Check sheet for the modelled part. Datum: model origin and axes. Units: mm. Face numbers are marked on the shaded views. A direction names the side the tool comes from. Round coordinates to 2 decimals unless told otherwise and drop trailing zeros. Order: outer loops, then holes, each group sorted by start corner. A loop starts at its lowest first (then second) coordinate and runs counter-clockwise, first axis right, second up. Notation, with made-up numbers: (85, -22.75) -> (140, -22.75) arc R10 ccw to (140, -14.75) -> close; hole circle Ø8 at (84.25, -8.5). An arc over 180 degrees is marked (long way). Answer in a Markdown table with one row per item.
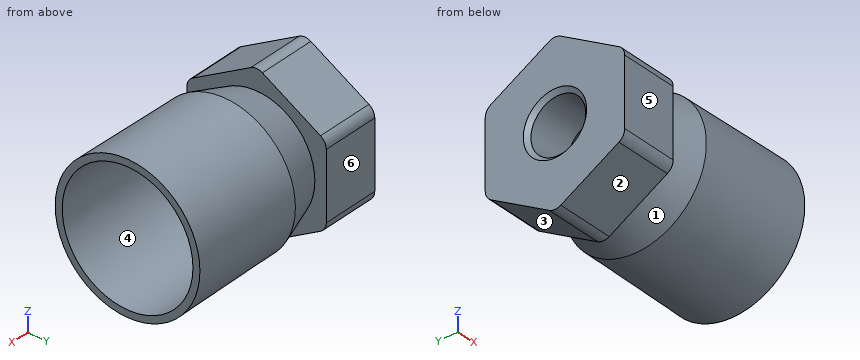
Autodesk Inventor part; units mm, degrees
ref_plane "YZ Plane" through (0, 0, 0) normal (1, 0, 0) x (0, 1, 0)
ref_plane "XZ Plane" through (0, 0, 0) normal (0, 1, 0) x (-1, 0, 0)
ref_plane "XY Plane" through (0, 0, 0) normal (0, 0, 1) x (1, 0, 0)
sketch "Sketch1" plane through (0, 0, 0) normal (0, 0, 1) x (1, 0, 0)
  line L0 (0, 0) -> (6.6144, 0) construction
  line L1 (0, 0) -> (0, 4.75) construction
  line L2 (0, 4.75) -> (8, 4.3864)
  line L3 (6.6144, 0) -> (16.6144, 0) construction
  line L4 (16.6144, 0) -> (16.6144, 12.2) construction
  line L5 (16.6144, 0) -> (36.6144, 0) construction
  line L6 (36.6144, 0) -> (36.6144, 12.45) construction
  line L7 (36.6144, 12.45) -> (16.6144, 12.2)
  line L8 (0, 4.75) -> (0, 6.75)
  line L9 (0, 4.75) -> (2, 4.75) construction
  line L10 (0, 6.75) -> (16.6144, 12.2)
  line L11 (8, 4.3864) -> (16.6144, 11)
  line L12 (16.6144, 11) -> (36.6144, 11.2499)
  line L13 (36.6144, 11.2499) -> (36.6144, 12.45)
  line L14 (0, 0) -> (3.3, 0) construction
  line L15 (3.3, 0) -> (3.3, 4.6) construction
  dimension "d2" = 4.75
  dimension "d3" = 12.2
  dimension "d4" = 20
  dimension "d5" = 12.45
  dimension "d6" = 2
  dimension "d7" = 90
  dimension "d8" = 1.2
  dimension "d9" = 1.2
  dimension "d10" = 10
  dimension "d24" = 177.397
  dimension "d25" = 8
  dimension "d26" = 3.3
  dimension "d27" = 4.6
  dimension "d28" = 6.6144
revolve "Revolution1" add sketch "Sketch1" angle 360 about axis through (6.6144, 0, 0) along (1, 0, 0)
sketch "Sketch2" plane through (0, 0, 0) normal (-1, 0, 0) x (0, 0, 1)
  circle A0 centre (0, 0) radius 6.75
  line L0 (0, -6.75) -> (0, -12.2) construction
  circle A1 centre (0, 0) radius 12.2
  line L1 (1.633, -6.5495) -> (2.9514, -11.8376)
  line L2 (-1.633, -6.5495) -> (-2.9514, -11.8376)
  point P0 (-1.633, -6.5495)
  point P1 (-2.9514, -11.8376)
  dimension "d12" = 14
extrude "Extrusion1" [suppressed]
chamfer "Chamfer1" [suppressed]
pattern_circular "Circular Pattern1" [suppressed]
chamfer "Chamfer2" distance 0.7 angle 45 1 edges at (0, -4.75, 0)
sketch "Sketch3" plane through (0, 0, 0) normal (-1, 0, 0) x (0, 0, 1)
  line L0 (-6.9282, -12) -> (-13.8564, 0)
  line L1 (-13.8564, 0) -> (-6.9282, 12)
  line L2 (-6.9282, 12) -> (6.9282, 12)
  line L3 (6.9282, 12) -> (13.8564, 0)
  line L4 (13.8564, 0) -> (6.9282, -12)
  line L5 (6.9282, -12) -> (-6.9282, -12)
  circle A0 centre (0, 0) radius 6.75
  point P0 (0, -12)
  dimension "d32" = 24
extrude "Extrusion2" add sketch "Sketch3" against normal blind 10
fillet "Fillet1" radius 2 6 edges at (5, 12, 6.9282) (5, 12, -6.9282) (5, 0, -13.8564) (5, -12, -6.9282) (5, -12, 6.9282) (5, 0, 13.8564)
equation "\"Tol\" = 0"
properties part number "PneumaticAdaptorFemale"
(1) Depth check by flat-ended pin: pin 1 Ø1.5 at (x, y) = (27, 2) entering from +Z; pin 2 Ø11 at (x, z) = (2.5, 1.5) entering from +Y; pin 3 Ø1 at (x, y) = (13.5, 4.5) entering from -Z. Enter the tip coordinate at first touch or a pass-through.
Solutions:
| item | result |
|---|---|
| pin 1 | z = 12.27 |
| pin 2 | y = 12 |
| pin 3 | z = -10.51 |
(2) Scan lines: probe 1 along Y at (x, z) = (26.5, 2.75); probe 2 along Y at (x, z) = (11, 4.5); probe 3 along Z at (x, y) = (27, -7.5). Record each from-to range of solid material in increasing order. Write a range as from..to.
Solutions:
| item | result |
|---|---|
| probe 1 | -12.01..-10.78, 10.78..12.01 |
| probe 2 | -9.33..-4.95, 4.95..9.33 |
| probe 3 | -9.79..-8.22, 8.22..9.79 |
(3) Section check A-A on x = 4. Record the boundary of the cut face in (y, z), plus the area to 3 significant figures.
Solutions:
| item | result |
|---|---|
| outline | (-12, -5.77) arc R2 ccw to (-11, -7.51) -> (-1, -13.28) arc R2 ccw to (1, -13.28) -> (11, -7.51) arc R2 ccw to (12, -5.77) -> (12, 5.77) arc R2 ccw to (11, 7.51) -> (1, 13.28) arc R2 ccw to (-1, 13.28) -> (-11, 7.51) arc R2 ccw to (-12, 5.77) -> close; hole circle Ø9.14 at (0, 0) |
| area | 432 mm^2 |
(4) Section check B-B on x = 10.5. Record the boundary of the cut face in (y, z), plus the area to 3 significant figures.
Solutions:
| item | result |
|---|---|
| outline | circle Ø20.39 at (0, 0); hole circle Ø12.61 at (0, 0) |
| area | 202 mm^2 |
(5) Draft check along Y on the marked faces 4, 5 and 6. Enter one of: pulls with the +Y half, pulls with the -Y half, needs draft (parallel to the pull), parting line crosses it, or undercut.
Solutions:
| item | result |
|---|---|
| face 4 | undercut |
| face 5 | pulls with the -Y half |
| face 6 | pulls with the +Y half |
(6) Tool access check on the marked faces 1, 2 and 3. Record the directions out of +Z, -Z, +X, -X, +Y, -Y that give a thin tool (end or side, any length) a straight path to the whole face; none if there is none.
Solutions:
| item | result |
|---|---|
| face 1 | none |
| face 2 | -Z, -X, -Y |
| face 3 | -Z, -X, +Y |
(7) Section check C-C on x = 24.5. Record the boundary of the cut face in (y, z), plus the area to 3 significant figures.
Solutions:
| item | result |
|---|---|
| outline | circle Ø24.6 at (0, 0); hole circle Ø22.2 at (0, 0) |
| area | 88.2 mm^2 |
